Geometry: final body of the model. Coordinates: model frame, mm. Coordinates: 2 decimals unless noted, no trailing zeros. Write each loop counter-clockwise with the first axis right and the second up, starting at its lowest first coordinate (ties: lowest second). Pieces come first, ordered by that corner, then holes.
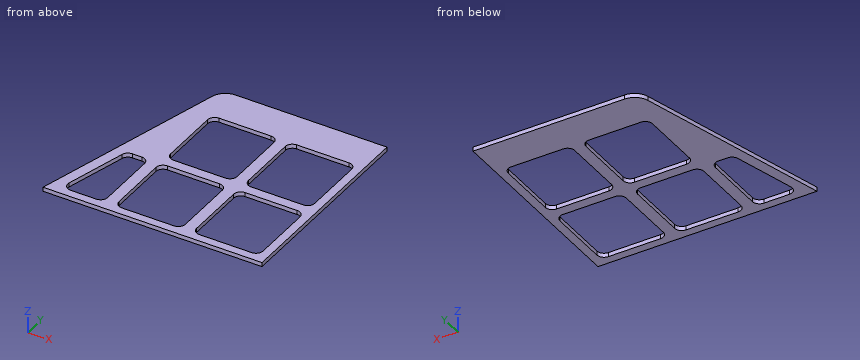
from build123d import *

# Parameters (mm, degrees)
BOSS_EXTRUDE1_DEPTH = 6.35
CUT_EXTRUDE1_DEPTH  = 6.35


with BuildPart() as part:
    # Sketch1 → Boss-Extrude1 (new body)
    with BuildSketch(Plane.XY):
        with BuildLine():
            Line((0, 0), (335.28, 0))
            Line((335.28, 0), (335.28, 313.51728))
            Line((335.28, 313.51728), (103.321320582, 313.51728))
            ThreePointArc((103.321320582, 313.51728), (87.853181888, 308.264157806), (78.783155215, 294.677648925))
            Line((78.783155215, 294.677648925), (0, 0))
        make_face()
    extrude(amount=BOSS_EXTRUDE1_DEPTH)

    # Sketch2 → Cut-Extrude1 (cut)
    with BuildSketch(Plane.XY.offset(6.35)):
        with BuildLine():
            Line((311.705446202, 12.7), (231.854553798, 12.7))
            ThreePointArc((231.854553798, 12.7), (224.165083065, 15.885083065), (220.98, 23.574553798))
            Line((220.98, 23.574553798), (220.98, 116.125446202))
            ThreePointArc((220.98, 116.125446202), (224.165083065, 123.814916935), (231.854553798, 127))
            Line((231.854553798, 127), (311.705446202, 127))
            ThreePointArc((311.705446202, 127), (319.394916935, 123.814916935), (322.58, 116.125446202))
            Line((322.58, 116.125446202), (322.58, 23.574553798))
            ThreePointArc((322.58, 23.574553798), (319.394916935, 15.885083065), (311.705446202, 12.7))
        make_face()
        with BuildLine():
            Line((203.603317785, 23.574553798), (203.603317785, 116.125446202))
            ThreePointArc((203.603317785, 116.125446202), (200.41823472, 123.814916935), (192.728763987, 127))
            Line((192.728763987, 127), (112.877871584, 127))
            ThreePointArc((112.877871584, 127), (105.18840085, 123.814916935), (102.003317785, 116.125446202))
            Line((102.003317785, 116.125446202), (102.003317785, 23.574553798))
            ThreePointArc((102.003317785, 23.574553798), (105.18840085, 15.885083065), (112.877871584, 12.7))
            Line((112.877871584, 12.7), (192.728763987, 12.7))
            ThreePointArc((192.728763987, 12.7), (200.41823472, 15.885083065), (203.603317785, 23.574553798))
        make_face()
        with BuildLine():
            Line((84.62663557, 23.574553798), (84.62663557, 116.125446202))
            ThreePointArc((84.62663557, 116.125446202), (81.441552505, 123.814916935), (73.752081772, 127))
            Line((73.752081772, 127), (59.157987156, 127))
            ThreePointArc((59.157987156, 127), (52.535581392, 124.750970083), (48.652412376, 118.934150328))
            Line((48.652412376, 118.934150328), (23.908590277, 26.383257925))
            ThreePointArc((23.908590277, 26.383257925), (25.788641176, 16.952148035), (34.414165057, 12.7))
            Line((34.414165057, 12.7), (73.752081772, 12.7))
            ThreePointArc((73.752081772, 12.7), (81.441552505, 15.885083065), (84.62663557, 23.574553798))
        make_face()
        with BuildLine():
            Line((203.603317785, 153.114553798), (203.603317785, 245.665446202))
            ThreePointArc((203.603317785, 245.665446202), (200.41823472, 253.354916935), (192.728763987, 256.54))
            Line((192.728763987, 256.54), (112.877871584, 256.54))
            ThreePointArc((112.877871584, 256.54), (105.18840085, 253.354916935), (102.003317785, 245.665446202))
            Line((102.003317785, 245.665446202), (102.003317785, 153.114553798))
            ThreePointArc((102.003317785, 153.114553798), (105.18840085, 145.425083065), (112.877871584, 142.24))
            Line((112.877871584, 142.24), (192.728763987, 142.24))
            ThreePointArc((192.728763987, 142.24), (200.41823472, 145.425083065), (203.603317785, 153.114553798))
        make_face()
        with BuildLine():
            Line((322.58, 153.114553798), (322.58, 245.665446202))
            ThreePointArc((322.58, 245.665446202), (319.394916935, 253.354916935), (311.705446202, 256.54))
            Line((311.705446202, 256.54), (231.854553798, 256.54))
            ThreePointArc((231.854553798, 256.54), (224.165083065, 253.354916935), (220.98, 245.665446202))
            Line((220.98, 245.665446202), (220.98, 153.114553798))
            ThreePointArc((220.98, 153.114553798), (224.165083065, 145.425083065), (231.854553798, 142.24))
            Line((231.854553798, 142.24), (311.705446202, 142.24))
            ThreePointArc((311.705446202, 142.24), (319.394916935, 145.425083065), (322.58, 153.114553798))
        make_face()
    extrude(amount=-CUT_EXTRUDE1_DEPTH, mode=Mode.SUBTRACT)


solid = part.part
Item 1: Section B-B, the plane y = 214. Output: boundary loops of the cut face in (x, z).
Derived:
outline: (57.21, 0) - (102, 0) - (102, 6.35) - (57.21, 6.35) - close; (203.6, 0) - (220.98, 0) - (220.98, 6.35) - (203.6, 6.35) - close; (322.58, 0) - (335.28, 0) - (335.28, 6.35) - (322.58, 6.35) - close
Item 2: Section D-D, the plane z = 3. State how many separate pieces and enclosed holes the cut face has, plus the area to 3 significant figures.
Derived:
separate pieces: 1
enclosed holes: 5
area: 40,400 mm2
Item 3: Section C-C, the plane x = 39. Output: boundary loops of the cut face in (y, z).
Derived:
outline: (0, 0) - (12.7, 0) - (12.7, 6.35) - (0, 6.35) - close; (82.83, 0) - (145.87, 0) - (145.87, 6.35) - (82.83, 6.35) - close
Item 4: Section A-A, the plane x = 140.5. Output: boundary loops of the cut face in (y, z).
Derived:
outline: (0, 0) - (12.7, 0) - (12.7, 6.35) - (0, 6.35) - close; (127, 0) - (142.24, 0) - (142.24, 6.35) - (127, 6.35) - close; (256.54, 0) - (313.52, 0) - (313.52, 6.35) - (256.54, 6.35) - close
Item 5: Pin query (flat end, axial travel): pin 1 (3 mm diameter, centred on y = 58, z = 2, fed in from -X). Return the tip coordinate at first contact, or that it passes through.
Derived:
pin 1: stops at x = 15.11
Item 6: Material intervals for probe 1 along Y at (x, z) = (141.5, 4.5); probe 2 along Y at (x, z) = (321, 3.25); probe 3 along X at (y, z) = (189, 3), sorted ascending.
Derived:
probe 1: y = 0 to 12.7, 127 to 142.24, 256.54 to 313.52
probe 2: y = 0 to 17.93, 121.77 to 147.47, 251.31 to 313.52
probe 3: x = 50.53 to 102, 203.6 to 220.98, 322.58 to 335.28
